```python
from build123d import *

# Parameters (mm, degrees)
BOSS_EXTRUDE1_DEPTH = 1.6
SKETCH2_W           = 8.7
SKETCH2_H           = 1
CUT_EXTRUDE1_DEPTH  = 1.6
SKETCH3_W           = 9.6
SKETCH3_H           = 1
BOSS_EXTRUDE2_DEPTH = 1.6


with BuildPart() as part:
    # Sketch1 → Boss-Extrude1 (new body)
    with BuildSketch(Plane.XY):
        Polygon((2.75, 0), (-2.75, 0), (-2.75, 1.5), (-13.95, 1.5), (-13.95, 11), (-4.35, 11), (-4.35, 9.5), (-3.25, 9.5), (-3.25, 3.1), (3.25, 3.1), (3.25, 9.5), (4.35, 9.5), (4.35, 11), (13.95, 11), (13.95, 1.5), (2.75, 1.5), align=None)
    extrude(amount=BOSS_EXTRUDE1_DEPTH)

    # Sketch2 → Cut-Extrude1 (cut)
    with BuildSketch(Plane.XY.offset(1.6)):
        with Locations((0, 9)):
            Rectangle(SKETCH2_W, SKETCH2_H)
    extrude(amount=-CUT_EXTRUDE1_DEPTH, mode=Mode.SUBTRACT)

    # Sketch3 → Boss-Extrude2 (add)
    with BuildSketch(Plane.XY.offset(1.6)):
        with Locations((-9.15, 11.5)):
            Rectangle(SKETCH3_W, SKETCH3_H)
        with Locations((9.15, 11.5)):
            Rectangle(SKETCH3_W, SKETCH3_H)
    extrude(amount=-BOSS_EXTRUDE2_DEPTH)


solid = part.part
```
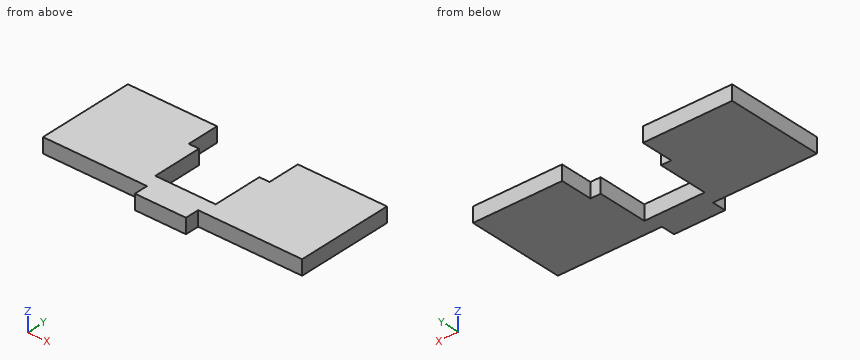
Design review of the part built by this model. Coordinates are the model's own, in mm. Give positions to 0.01 mm unless a question says otherwise; leave off trailing zeros. Loops run counter-clockwise (first coordinate to the right, second up) from the corner with the lowest first, then second, coordinate; pieces in that order, holes last. Notation, with made-up numbers: M -34.75,-17 L -23.75,-17 A27 cw -23.75,16 Z; hole C 82,80 d8. An arc over 180 degrees is marked long. Return JSON: item names as keys, results as strings. Group by question number.
Item 1: For probe 1 along X at (y, z) = (9.25, 1.2); probe 2 along X at (y, z) = (4, 1.05); probe 3 along Y at (x, z) = (-8, 1.2), list the stretches that pass through material, from the lowest coordinate up.
Item 2: We need section C-C (y = 6.5). Give the boundary of the cut face in (x, z).
Item 3: We need section A-A (y = 9.75). Give the boundary of the cut face in (x, z), and give its area (3 significant figures).
Item 4: Insertion check: pin 1 Ø0.8 at (y, z) = (1, 0.5) entering from -X; pin 2 Ø0.8 at (x, z) = (-1, 1) entering from +Y; pin 3 Ø0.5 at (x, z) = (-4, 0.5) entering from +Y. Each pin has a flat end and moves straight along its axis. Give the tip position at first contact, or say it passes through.
Item 5: We need section B-B (z = 0.8). Give the boundary of the cut face in (x, y), and give its area (3 significant figures).
Item 6: We need section D-D (x = -3.75). Give the boundary of the cut face in (y, z).
Output:
{
 "1": {"probe 1": "x = -13.95 to -4.35, 4.35 to 13.95", "probe 2": "x = -13.95 to -3.25, 3.25 to 13.95", "probe 3": "y = 1.5 to 12"},
 "2": {"outline": "M -13.95,0 L -3.25,0 L -3.25,1.6 L -13.95,1.6 Z; M 3.25,0 L 13.95,0 L 13.95,1.6 L 3.25,1.6 Z"},
 "3": {"outline": "M -13.95,0 L -4.35,0 L -4.35,1.6 L -13.95,1.6 Z; M 4.35,0 L 13.95,0 L 13.95,1.6 L 4.35,1.6 Z", "area": "30.7 mm^2"},
 "4": {"pin 1": "stops at x = -2.75", "pin 2": "stops at y = 3.1", "pin 3": "stops at y = 8.5"},
 "5": {"outline": "M -13.95,1.5 L -2.75,1.5 L -2.75,0 L 2.75,0 L 2.75,1.5 L 13.95,1.5 L 13.95,12 L 4.35,12 L 4.35,8.5 L 3.25,8.5 L 3.25,3.1 L -3.25,3.1 L -3.25,8.5 L -4.35,8.5 L -4.35,12 L -13.95,12 Z", "area": "236 mm^2"},
 "6": {"outline": "M 1.5,0 L 8.5,0 L 8.5,1.6 L 1.5,1.6 Z"}
}
